Geometry: final body of the model. Coordinates: model frame, mm. Face numbers are marked on the shaded views. A direction names the side the tool comes from. Give positions to 0.01 mm unless a question says otherwise; leave off trailing zeros. Order: outer loops, then holes, each group sorted by start corner. A loop starts at its lowest first (then second) coordinate and runs counter-clockwise, first axis right, second up. Notation, with made-up numbers: (8, -6.5) - (21, -6.5) arc R13 ccw to (21, -0.5) - close; hole circle Ø7 at (81, 13.25). An arc over 180 degrees is marked (long way). Put each result on its own line as item: value. Start each with the question number.
1. First-contact query: P1, Ø4, axis at x = -10.3, z = 6, coming from the -Y side; P2, Ø5, axis at y = -1.5, z = 4, coming from the +X side; P3, Ø3, axis at x = 13.5, z = 8.5, coming from the -Y side. Flat tips, straight axial feed; report the tip coordinate or a pass-through.
2. Section D-D on z = 2.25. Return the cut outline in (x, y).
3. Section A-A on x = 0. Return the cut outline in (y, z).
4. Section B-B on y = -3.25. Return the cut outline in (x, z), plus the area to 3 significant figures.
5. Section C-C on x = 9. Return the cut outline in (y, z).
6. Set-up query: the marked faces 4, 5 and 6. Return all of +Z, -Z, +X, -X, +Y, -Y with unobstructed straight access to the full face (end or side cutting, diameter ignored); none if empty.
7. Ray query, line 1 along Z through (x, y) = (9.5, 3.25); line 2 along Y through (x, z) = (15.5, 5); line 3 along Z through (x, y) = (13.5, -8.45). Return the intervals inside material, ascending. Write a range as from..to.
8. Mould query, pull axis X, two halves, no side actions, for the marked faces 1, 2 and 3. Classes: pulls with the +X half, pulls with the -X half, needs draft (parallel to the pull), parting line crosses it, or undercut.
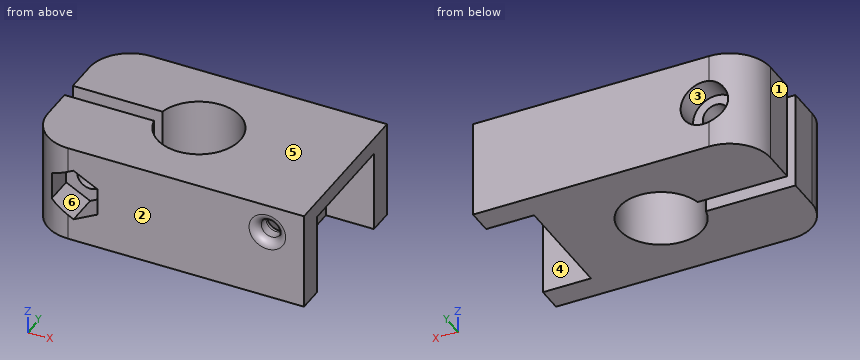
from build123d import *

# Parameters (mm, degrees)
F1_DEPTH     = 12
F2_W         = 5.9
F2_H         = 13.7
F3_DEPTH     = 10
F4_R         = 1.6
F5_DEPTH     = 20.001
F6_R         = 1.25
F7_DEPTH     = 16
F9_R         = 0.95
F10_DEPTH    = 7
F11_R        = 1.6
F12_DEPTH    = 4
F13_R        = 2.8
F14_DEPTH    = 3
F15_T1_DEPTH = 37


# Not quite as in the source:
# - a fillet or chamfer that OpenCascade refuses, or shapes differently, is made with other operations: its cross-section is extruded or revolved along the edge and cut away or added


with BuildPart() as f1:
    # F0 (on Top) → F1 (new body)
    with BuildSketch(Plane.XY):
        with BuildLine():
            Line((18, 10), (-16, 10))
            Line((-16, 10), (-16, 1))
            Line((-16, 1), (-5.0009999, 1))
            ThreePointArc((-5.0009999, 1), (5.1, 0), (-5.0009999, -1))
            Line((-5.0009999, -1), (-16, -1))
            Line((-16, -1), (-16, -10))
            Line((-16, -10), (18, -10))
            Line((18, -10), (18, -6.85))
            Line((18, -6.85), (18, 6.85))
            Line((18, 6.85), (18, 10))
        make_face()
    extrude(amount=F1_DEPTH)

    # F2 (on face) → F3 (cut)
    with BuildSketch(Plane(origin=(0, 0, 0), x_dir=(1, 0, 0), z_dir=(0, 0, -1))):
        with Locations((15.05, 0)):
            Rectangle(F2_W, F2_H)
    extrude(amount=-F3_DEPTH, mode=Mode.SUBTRACT)

    # F4 (on face) → F5 (cut, through all)
    with BuildSketch(Plane.XZ.offset(10)):
        with Locations((-10.3, 6)):
            Circle(F4_R)
    extrude(amount=-F5_DEPTH, mode=Mode.SUBTRACT)

    # F6 (on face) → F7 (cut)
    with BuildSketch(Plane.XZ.offset(10)):
        with Locations((13.5, 8.5)):
            Circle(F6_R)
    extrude(amount=-F7_DEPTH, mode=Mode.SUBTRACT)

    # F8: fillet of radius 1 on 2 edges, made by hand

    # F8_s1 → F8_t2 (revolve, cut)
    with BuildSketch(Plane.XY.offset(8.5)):
        with BuildLine():
            ThreePointArc((15.75, -10), (15.0428932188, -9.7071067812), (14.75, -9))
            Line((14.75, -9), (14.75, -10))
            Line((14.75, -10), (15.75, -10))
        make_face()
    revolve(axis=Axis((13.5, -10, 8.5), (0, -1, 0)), mode=Mode.SUBTRACT)


with BuildPart() as f8_tool4:
    # F8_s5 → F8_t6 (revolve)
    with BuildSketch(Plane.XY.offset(8.5)):
        with BuildLine():
            ThreePointArc((15.75, -6.85), (15.0428932188, -7.1428932188), (14.75, -7.85))
            Line((14.75, -7.85), (14.75, -6.85))
            Line((14.75, -6.85), (15.75, -6.85))
        make_face()
    revolve(axis=Axis((13.5, -6.85, 8.5), (0, -1, 0)))

    split(bisect_by=Plane.XY.offset(10), keep=Keep.BOTTOM)

    split(bisect_by=Plane.YZ.offset(12.1), keep=Keep.TOP)


with BuildPart() as f1_1:
    add(f1.part)

    # F8_t3: cut F8_tool4
    add(f8_tool4.part, mode=Mode.SUBTRACT)

    # F9 (on face) → F10 (cut)
    with BuildSketch(Plane.YZ.offset(12.1)):
        with Locations((46.374425292, 0.8309943862)):
            Circle(F9_R)
        with Locations((46.374425292, -5.6690056138)):
            Circle(F9_R)
        with Locations((-3.25, 5)):
            Circle(F9_R)
        with Locations((3.25, 5)):
            Circle(F9_R)
    extrude(amount=-F10_DEPTH, mode=Mode.SUBTRACT)

    # F11 (on face) → F12 (cut)
    with BuildSketch(Plane.XZ.offset(10)):
        Polygon((-7.35, 7.6736242323), (-10.3143082515, 9.227305642), (-13.25, 7.6886229858), (-13.25, 4.3268273558), (-10.3, 2.7806453228), (-7.35, 4.3268273558), align=None)
        with Locations((-10.3, 6)):
            Circle(F11_R, mode=Mode.SUBTRACT)
    extrude(amount=-F12_DEPTH, mode=Mode.SUBTRACT)

    # F13 (on face) → F14 (cut)
    with BuildSketch(Plane(origin=(0, 10, 0), x_dir=(-1, 0, 0), z_dir=(0, 1, 0))):
        with Locations((10.3, 6)):
            Circle(F13_R)
    extrude(amount=-F14_DEPTH, mode=Mode.SUBTRACT)

    # F15: fillet of radius 5 on 2 edges, made by hand

    # F15_s2 → F15_t1 (cut)
    with BuildSketch(Plane.XY.offset(-12.5)):
        with BuildLine():
            ThreePointArc((-11, -10), (-14.5355339059, -8.5355339059), (-16, -5))
            Line((-16, -5), (-16, -10))
            Line((-16, -10), (-11, -10))
        make_face()
        with BuildLine():
            ThreePointArc((-11, 10), (-14.5355339059, 8.5355339059), (-16, 5))
            Line((-16, 5), (-16, 10))
            Line((-16, 10), (-11, 10))
        make_face()
    extrude(amount=F15_T1_DEPTH, mode=Mode.SUBTRACT)


solid = f1_1.part
Resolved:
1. P1: y = -6
1. P2: x = 12.1
1. P3: y = -9.66
2. outline: (-16, -5) arc R5 ccw to (-11, -10) - (18, -10) - (18, -6.85) - (12.1, -6.85) - (12.1, 6.85) - (18, 6.85) - (18, 10) - (-11, 10) arc R5 ccw to (-16, 5) - (-16, 1) - (-5, 1) arc R5.1 cw (long way) to (-5, -1) - (-16, -1) - close
3. outline: (-10, 0) - (-5.1, 0) - (-5.1, 12) - (-10, 12) - close; (5.1, 0) - (10, 0) - (10, 12) - (5.1, 12) - close
4. outline: (-16, 0) - (-3.93, 0) - (-3.93, 12) - (-16, 12) - close; (3.93, 0) - (12.1, 0) - (12.1, 4.05) - (5.1, 4.05) - (5.1, 5.95) - (12.1, 5.95) - (12.1, 10) - (18, 10) - (18, 12) - (3.93, 12) - close; hole circle Ø3.2 at (-10.3, 6)
4. area: 233 mm^2
5. outline: (-10, 0) - (10, 0) - (10, 12) - (-10, 12) - close; hole circle Ø1.9 at (-3.25, 5); hole circle Ø1.9 at (3.25, 5)
6. face 4: -Z, +X
6. face 5: +Z, +X, -X, +Y, -Y
6. face 6: -Y
7. line 1: 0..4.05, 5.95..12
7. line 2: -10..-6.85, 6.85..10
7. line 3: 0..7.25, 9.75..12
8. face 1: pulls with the -X half
8. face 2: needs draft
8. face 3: undercut
